from build123d import *

# Parameters (mm, degrees)
F0_W     = 30
F0_H     = 40
F1_DEPTH = 24
F2_W     = 25
F2_H     = 40
F3_DEPTH = 20
F4_R     = 2.4
F5_DEPTH = 1.6


with BuildPart() as f1:
    # F0 (on Top) → F1 (new body)
    with BuildSketch(Plane.XY):
        Rectangle(F0_W, F0_H)
    extrude(amount=F1_DEPTH)

    # F2 (on face) → F3 (cut)
    with BuildSketch(Plane.XY.offset(24)):
        with Locations((2.5, 0)):
            Rectangle(F2_W, F2_H)
    extrude(amount=-F3_DEPTH, mode=Mode.SUBTRACT)

    # F4 (on face) → F5 (join)
    with BuildSketch(Plane(origin=(-15, 0, 0), x_dir=(0, -1, 0), z_dir=(-1, 0, 0))):
        with Locations((-16, 4)):
            Circle(F4_R)
        with Locations((-16, 12)):
            Circle(F4_R)
        with Locations((-16, 20)):
            Circle(F4_R)
        with Locations((-8, 4)):
            Circle(F4_R)
        with Locations((-8, 12)):
            Circle(F4_R)
        with Locations((-8, 20)):
            Circle(F4_R)
        with Locations((0, 4)):
            Circle(F4_R)
        with Locations((0, 12)):
            Circle(F4_R)
        with Locations((0, 20)):
            Circle(F4_R)
        with Locations((8, 4)):
            Circle(F4_R)
        with Locations((8, 12)):
            Circle(F4_R)
        with Locations((8, 20)):
            Circle(F4_R)
        with Locations((16, 4)):
            Circle(F4_R)
        with Locations((16, 12)):
            Circle(F4_R)
        with Locations((16, 20)):
            Circle(F4_R)
    extrude(amount=F5_DEPTH)


solid = f1.part
Build history of the part. All positions in model axes, mm. A direction names the side the tool comes from. Coordinates: 2 decimals unless noted, no trailing zeros. Write each loop counter-clockwise with the first axis right and the second up, starting at its lowest first coordinate (ties: lowest second). Pieces come first, ordered by that corner, then holes.
(1) Cut at C-C on x = 13.5. List the corners of the cut face in (y, z), and give its area (3 significant figures).
(2) Mould opens along Y. For faces 4 (the flat face through (-16.6, 16, 20)), 5 (the cylindrical face through (-15.789, 0.52, 17.657)), 6 (the cylindrical face through (-15.789, -13.602, 12.106)) say: pulls with the +Y half, pulls with the -Y half, needs draft (parallel to the pull), parting line crosses it, or undercut.
(3) Cut at A-A on y = -16. List the corners of the cut face in (x, z), and give its area (3 significant figures).
(4) 3-axis set-ups, long thin cutter, end or side, ignore diameter. For faces 1 (the flat face through (-16.6, 16, 12)), 2 (the flat face through (-10, 0, 14)), 3 (the cylindrical face through (-15.789, 18.398, 12.106)): which of +Z, -Z, +X, -X, +Y, -Y reach the whole face in a straight line?
(5) Cut at D-D on z = 7.25. List the corners of the cut face in (x, y).
(6) Cut at B-B on z = 20. List the corners of the cut face in (x, y), and give its area (3 significant figures).
(7) Drill centre lines: line 1 (X direction, y = 4, z = 7.75); line 2 (Z direction, x = -0.5, y = -15.5); line 3 (X direction, y = -4, z = 1). Where is each one in solid material? Low to high.
(8) Pin check, flat tips, straight feed: pin 1 Ø6 at (y, z) = (5, 15.5) entering from +X; pin 2 Ø5 at (y, z) = (-3, 9) entering from -X. Stop position of each tip, or through.
Working result:
1. outline: (-20, 0) - (20, 0) - (20, 4) - (-20, 4) - close
1. area: 160 mm2
2. face 4: needs draft
2. face 5: undercut
2. face 6: undercut
3. outline: (-16.6, 1.6) - (-15, 1.6) - (-15, 0) - (15, 0) - (15, 4) - (-10, 4) - (-10, 24) - (-15, 24) - (-15, 22.4) - (-16.6, 22.4) - (-16.6, 17.6) - (-15, 17.6) - (-15, 14.4) - (-16.6, 14.4) - (-16.6, 9.6) - (-15, 9.6) - (-15, 6.4) - (-16.6, 6.4) - close
3. area: 243 mm2
4. face 1: +Z, -Z, -X, +Y, -Y
4. face 2: +Z, +X, +Y, -Y
4. face 3: -X
5. outline: (-15, -20) - (-10, -20) - (-10, 20) - (-15, 20) - close
6. outline: (-16.6, -18.4) - (-15, -18.4) - (-15, -20) - (-10, -20) - (-10, 20) - (-15, 20) - (-15, 18.4) - (-16.6, 18.4) - (-16.6, 13.6) - (-15, 13.6) - (-15, 10.4) - (-16.6, 10.4) - (-16.6, 5.6) - (-15, 5.6) - (-15, 2.4) - (-16.6, 2.4) - (-16.6, -2.4) - (-15, -2.4) - (-15, -5.6) - (-16.6, -5.6) - (-16.6, -10.4) - (-15, -10.4) - (-15, -13.6) - (-16.6, -13.6) - close
6. area: 238 mm2
7. line 1: x = -15 to -10
7. line 2: z = 0 to 4
7. line 3: x = -15 to 15
8. pin 1: stops at x = -10
8. pin 2: stops at x = -16.6
